Could you check a few things on this model? Use its own coordinates, in mm. Round coordinates to 2 decimals unless told otherwise and drop trailing zeros. Write each loop counter-clockwise with the first axis right and the second up, starting at its lowest first coordinate (ties: lowest second). Pieces come first, ordered by that corner, then holes. Notation, with made-up numbers: (81, 7) -> (125, 7) arc R13 ccw to (125, 31) -> close; hole circle Ø5 at (60.5, 66.5). An arc over 180 degrees is marked (long way). Return JSON: item names as keys, results as strings.
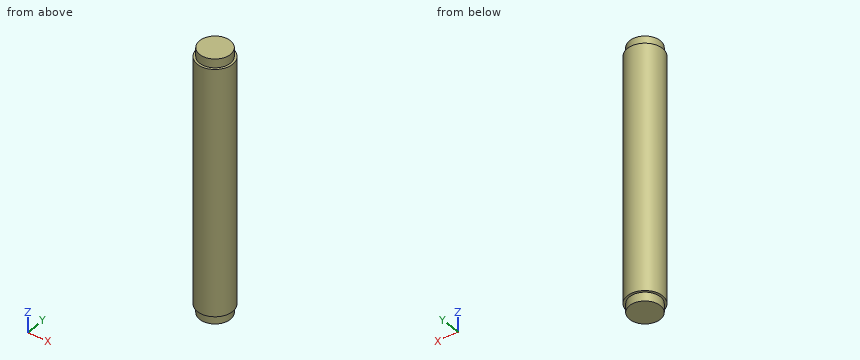
from build123d import *

# Parameters (mm, degrees)
BOSS_EXTRUDE1_START = 190.5
SKETCH1_R           = 25.4
BOSS_EXTRUDE1_DEPTH = 381
SKETCH2_R           = 25.4
SKETCH2_R_2         = 22.225
CUT_EXTRUDE1_DEPTH  = 12.7
CUT_EXTRUDE2_START  = -12.7
SKETCH3_R           = 25.4
SKETCH3_R_2         = 22.225
CUT_EXTRUDE2_DEPTH  = 12.7


with BuildPart() as part:
    # Sketch1 → Boss-Extrude1 (new body)
    with BuildSketch(Plane.XY.offset(BOSS_EXTRUDE1_START)):
        Circle(SKETCH1_R)
    extrude(amount=-BOSS_EXTRUDE1_DEPTH)

    # Sketch2 → Cut-Extrude1 (cut)
    with BuildSketch(Plane.XY.offset(190.5)):
        Circle(SKETCH2_R)
        Circle(SKETCH2_R_2, mode=Mode.SUBTRACT)
    extrude(amount=-CUT_EXTRUDE1_DEPTH, mode=Mode.SUBTRACT)

    # Sketch3 → Cut-Extrude2 (cut)
    with BuildSketch(Plane(origin=(0, 0, -190.5), x_dir=(-1, 0, 0), z_dir=(0, 0, -1)).offset(CUT_EXTRUDE2_START)):
        with Locations(Location((0, 0, 0), (0, 0, 180))):
            Circle(SKETCH3_R)
        with Locations(Location((0, 0, 0), (0, 0, 180))):
            Circle(SKETCH3_R_2, mode=Mode.SUBTRACT)
    extrude(amount=CUT_EXTRUDE2_DEPTH, mode=Mode.SUBTRACT)


solid = part.part
1) If I drill on probe 1 along Y at (x, z) = (0.5, -23); probe 2 along Z at (x, y) = (-17.5, 14); probe 3 along X at (y, z) = (20.5, 18.5), over which ranges is the centre line in solid material (lowest first)? Write a range as [from, to].
Return value:
{"probe 1": "[-25.4, 25.4]", "probe 2": "[-177.8, 177.8]", "probe 3": "[-15, 15]"}
2) I want a section at A-A, the plane y = 5.5. Please give me the cut outline in (x, z), and give its area (3 significant figures).
Return value:
{"outline": "(-24.8, -177.8) -> (-21.53, -177.8) -> (-21.53, -190.5) -> (21.53, -190.5) -> (21.53, -177.8) -> (24.8, -177.8) -> (24.8, 177.8) -> (21.53, 177.8) -> (21.53, 190.5) -> (-21.53, 190.5) -> (-21.53, 177.8) -> (-24.8, 177.8) -> close", "area": "18,700 mm²"}
3) Will these pins go through, and if not, where does the flat tip stop? pin 1 Ø6 at (x, z) = (-9, 113.5) entering from -Y; pin 2 Ø10 at (x, z) = (12, -72.5) entering from -Y; pin 3 Ø1.5 at (x, y) = (-19.5, 12.5) entering from -Z.
Return value:
{"pin 1": "y = -24.68", "pin 2": "y = -24.42", "pin 3": "z = -177.8"}
4) I want a section at B-B, the plane x = -6.5. Please give me the cut outline in (y, z), and give its area (3 significant figures).
Return value:
{"outline": "(-24.55, -177.8) -> (-21.25, -177.8) -> (-21.25, -190.5) -> (21.25, -190.5) -> (21.25, -177.8) -> (24.55, -177.8) -> (24.55, 177.8) -> (21.25, 177.8) -> (21.25, 190.5) -> (-21.25, 190.5) -> (-21.25, 177.8) -> (-24.55, 177.8) -> close", "area": "18,500 mm²"}
5) I want a section at C-C, the plane z = 4. Please give me the cut outline in (x, y).
Return value:
{"outline": "circle Ø50.8 at (0, 0)"}
